For this review, take the finished solid that the model builds, in its own axes (mm). A direction names the side the tool comes from. Coordinates: 2 decimals unless noted, no trailing zeros. Loops run counter-clockwise (first coordinate to the right, second up) from the corner with the lowest first, then second, coordinate; pieces in that order, holes last.
1. Machinability: for faces 4 (the face through (46, 12.7, 5)), 5 (the face through (44.22, 11.135, -12.645)), 6 (the face through (-1.64, 11.13, -45.96)), which of the approach directions +Z, -Z, +X, -X, +Y, -Y give a long, thin tool a straight path to every point of the face, cutting with its end or side? Answer none if there is none.
2. Mouldability with a two-part tool opening along Z and no side actions: class faces 1 (the face through (35.254, 11.135, 29.538)), 2 (the face through (-19, 12.7, 42)), 3 (the face through (7.954, 11.135, -45.3)) as pulls with the +Z half, pulls with the -Z half, needs draft (parallel to the pull), parting line crosses it, or undercut.
3. Clearance check with flat-ended pins moving along their axes: P1, Ø7.5, axis at x = 33.5, z = 30.5, coming from the +Y side; P2, Ø5, axis at x = 12.5, y = 3.5, coming from the +Z side; P3, Ø9, axis at x = 0, z = 0, coming from the -Y side; P4, Ø1, axis at x = 45, y = 12, coming from the -Z side. State where each tip first meets the part, or that it passes through.
4. Take a section at D-D, the plane y = 23. State the section outline as (x, z) points (3 decimals), then the cut area to 3 significant figures.
5. To check wall thickness, follow probe 1 along Z at (x, y) = (0, 1); probe 2 along X at (y, z) = (11.25, -17); probe 3 along Z at (x, y) = (0, 20.75) (3 decimals). State the ranges of each line that lie inside material, in increasing order.
6. Take a section at C-C, the plane y = 18. State the section outline as (x, z) points (3 decimals).
```python
from build123d import *

# Parameters (mm, degrees)
SKETCH2_W          = 12.7
SKETCH2_H          = 6.35
CUT_EXTRUDE1_DEPTH = 3.175
CIRPATTERN1_COUNT  = 30


with BuildPart() as part:
    # Sketch1 → Revolve1 (revolve)
    with BuildSketch(Plane.XY):
        Polygon((-7.62, 0), (-46.0375, 0), (-46.0375, 1.2065), (-43.4975, 1.2065), (-43.4975, 4.7625), (-46.0375, 4.7625), (-46.0375, 6.35), (-49.2125, 6.35), (-49.2125, 12.7), (-42.8625, 12.7), (-42.8625, 9.525), (-33.02, 9.525), (-17.145, 25.4), (-13.97, 25.4), (-13.97, 9.525), (-7.62, 3.175), align=None)
    revolve(axis=Axis((0, -42.3, 0), (0, 1, 0)))

    # Sketch2 → Cut-Extrude1 (cut)
    with BuildSketch(Plane(origin=(0, 12.7, 0), x_dir=(1, 0, 0), z_dir=(0, 1, 0))):
        with Locations((49.094745657, 0)):
            Rectangle(SKETCH2_W, SKETCH2_H)
    cut_extrude1 = extrude(amount=-CUT_EXTRUDE1_DEPTH, mode=Mode.SUBTRACT)

    # CirPattern1: Cut-Extrude1 ×30 about axis
    cirpattern1_axis = Axis((0, 0, 0), (0, 1, 0))
    for i in range(1, CIRPATTERN1_COUNT):
        add(cut_extrude1.rotate(cirpattern1_axis, i * 360 / CIRPATTERN1_COUNT), mode=Mode.SUBTRACT)


solid = part.part
```
Results list:
1. face 4: +Z, -Z, +X, +Y
1. face 5: +X, +Y
1. face 6: +Y
2. face 1: undercut
2. face 2: needs draft
2. face 3: pulls with the -Z half
3. P1: stops at y = 12.7
3. P2: stops at z = 44.86
3. P3: passes through
3. P4: stops at z = -16.78
4. outline: circle Ø39.09 at (0, 0); hole circle Ø27.94 at (0, 0)
4. area: 587 mm2
5. probe 1: z = -46.04 to -7.62, 7.62 to 46.04
5. probe 2: x = -46.18 to -45.99, -26.28 to 26.28, 45.99 to 46.18
5. probe 3: z = -21.795 to -13.97, 13.97 to 21.795
6. outline: circle Ø49.09 at (0, 0); hole circle Ø27.94 at (0, 0)
